CAD build for the part. Positions are in the model's coordinates, mm. Give positions to 0.01 mm unless a question says otherwise; leave off trailing zeros. Write each loop counter-clockwise with the first axis right and the second up, starting at its lowest first coordinate (ties: lowest second). Pieces come first, ordered by that corner, then holes. Notation, with made-up numbers: (42, 45.25) -> (65, 45.25) arc R28 cw to (65, 75.25) -> close; hole circle Ø3 at (62.5, 32). An arc over 180 degrees is marked (long way). Answer as a JSON object with one key per item and string values.
```python
from build123d import *

# Parameters (mm, degrees)
F0_R          = 15.685168
F1_DEPTH      = 25.4
F1_DEPTH_BACK = 25.4
F3_DEPTH      = 6.35
F5_R          = 5.939538
F6_DEPTH      = 50.801


with BuildPart() as f1:
    # F0 (on Front) → F1 (new body, two sides)
    with BuildSketch(Plane.XZ) as f1_sk:
        Circle(F0_R)
    extrude(amount=F1_DEPTH)
    extrude(f1_sk.sketch, amount=-F1_DEPTH_BACK)

    # F2 (on face) → F3 (join)
    with BuildSketch(Plane.XZ.offset(25.4)):
        with BuildLine():
            Line((-15.685168, 37.850551), (-15.685168, 0))
            ThreePointArc((-15.685168, 0), (0, -15.685168), (15.685168, 0))
            Line((15.685168, 0), (15.685168, 37.850551))
            ThreePointArc((15.685168, 37.850551), (11.091089, 48.94164), (0, 53.53572))
            ThreePointArc((0, 53.53572), (-11.091089, 48.94164), (-15.685168, 37.850551))
        make_face()
    extrude(amount=-F3_DEPTH)

    # F4: F1 across plane


with BuildPart() as f1_1:
    add(f1.part)
    add(f1.part.mirror(Plane.XZ))

    # F5 (on face) → F6 (cut, through all)
    with BuildSketch(Plane.XZ.offset(25.4)):
        with Locations((0, 37.850551)):
            Circle(F5_R)
        Circle(F5_R)
    extrude(amount=-F6_DEPTH, mode=Mode.SUBTRACT)


solid = f1_1.part
```
1) Slice it at A-A (y = 21). List the corners of the cut face in (x, z).
Model answer:
{"outline": "(-15.69, 0) arc R15.69 ccw to (15.69, 0) -> (15.69, 37.85) arc R15.69 ccw to (0, 53.54) arc R15.69 ccw to (-15.69, 37.85) -> close; hole circle Ø11.88 at (0, 0); hole circle Ø11.88 at (0, 37.85)"}
2) Pin check, flat tips, straight feed: pin 1 (6 mm diameter, centred on x = 9, y = -1.5, fed in from +Z); pin 2 (4 mm diameter, centred on x = -9.5, y = 14, fed in from -Z); pin 3 (10 mm diameter, centred on x = 4, y = 8.5, fed in from +Z). Stop position of each tip, or through.
Model answer:
{"pin 1": "stops at z = 14.49", "pin 2": "stops at z = -13.78", "pin 3": "stops at z = 15.69"}
3) Mould opens along Z. For faces 1 (the cylindrical face through (-3.4, -0.356, -15.312)), 2 (the cylindrical face through (3.19, 22.18, 42.86)), 3 (the flat face through (15.685, -22, 19)) say: released by +Z, released by -Z, zero draft, split by the parting line, or undercut.
Model answer:
{"face 1": "split by the parting line", "face 2": "undercut", "face 3": "zero draft"}
4) Slice it at D-D (x = -12). List the corners of the cut face in (y, z), then the cut area to 3 significant figures.
Model answer:
{"outline": "(-25.4, -10.1) -> (25.4, -10.1) -> (25.4, 47.95) -> (19.05, 47.95) -> (19.05, 10.1) -> (-19.05, 10.1) -> (-19.05, 47.95) -> (-25.4, 47.95) -> close", "area": "1,510 mm2"}
5) Slice it at B-B (x = 3.5). List the corners of the cut face in (y, z), then the cut area to 3 significant figures.
Model answer:
{"outline": "(-25.4, -15.29) -> (25.4, -15.29) -> (25.4, -4.8) -> (-25.4, -4.8) -> close; (-25.4, 4.8) -> (25.4, 4.8) -> (25.4, 33.05) -> (19.05, 33.05) -> (19.05, 15.29) -> (-19.05, 15.29) -> (-19.05, 33.05) -> (-25.4, 33.05) -> close; (-25.4, 42.65) -> (-19.05, 42.65) -> (-19.05, 53.14) -> (-25.4, 53.14) -> close; (19.05, 42.65) -> (25.4, 42.65) -> (25.4, 53.14) -> (19.05, 53.14) -> close", "area": "1,420 mm2"}
6) Slice it at C-C (z = 41). List the corners of the cut face in (x, y), then the cut area to 3 significant figures.
Model answer:
{"outline": "(-15.37, -25.4) -> (-5.04, -25.4) -> (-5.04, -19.05) -> (-15.37, -19.05) -> close; (-15.37, 19.05) -> (-5.04, 19.05) -> (-5.04, 25.4) -> (-15.37, 25.4) -> close; (5.04, -25.4) -> (15.37, -25.4) -> (15.37, -19.05) -> (5.04, -19.05) -> close; (5.04, 19.05) -> (15.37, 19.05) -> (15.37, 25.4) -> (5.04, 25.4) -> close", "area": "262 mm2"}
7) Wall check: probe 1 along Z at (x, y) = (0, -22); probe 2 along Z at (x, y) = (0, -11.5); probe 3 along Y at (x, z) = (4.5, 33.5). Give the ranges that are in metal, low to high.
Model answer:
{"probe 1": "z = -15.69 to -5.94, 5.94 to 31.91, 43.79 to 53.54", "probe 2": "z = -15.69 to -5.94, 5.94 to 15.69", "probe 3": "y = -25.4 to -19.05, 19.05 to 25.4"}
